```python
from build123d import *

# Parameters (mm, degrees)
F1_DEPTH = 25.4


with BuildPart() as f1:
    # F0 (on Front) → F1 (new body)
    with BuildSketch(Plane.XZ):
        with BuildLine():
            Line((6.3292504433, 31.1127480115), (4.2333333333, 31.4665121818))
            ThreePointArc((4.2333333333, 31.4665121818), (-31.75, 0), (4.2333333333, -31.4665121818))
            Line((4.2333333333, -31.4665121818), (6.3292504433, -31.1127480115))
            ThreePointArc((6.3292504433, -31.1127480115), (24.5867464457, -20.0886634501), (31.75, 0))
            ThreePointArc((31.75, 0), (24.5867464457, 20.0886634501), (6.3292504433, 31.1127480115))
        make_face()
        with BuildLine():
            Line((25.4, 5.588), (25.4, 0))
            Line((25.4, 0), (25.4, -5.588))
            Line((25.4, -5.588), (11.4045717149, -5.588))
            ThreePointArc((11.4045717149, -5.588), (0, -12.7), (-11.4045717149, -5.588))
            Line((-11.4045717149, -5.588), (-25.4, -5.588))
            Line((-25.4, -5.588), (-25.4, 5.588))
            Line((-25.4, 5.588), (-11.4045717149, 5.588))
            ThreePointArc((-11.4045717149, 5.588), (0, 12.7), (11.4045717149, 5.588))
            Line((11.4045717149, 5.588), (25.4, 5.588))
        make_face(mode=Mode.SUBTRACT)
        with BuildLine():
            Line((79.3705518859, 18.7843046381), (6.3292504433, 31.1127480115))
            ThreePointArc((6.3292504433, 31.1127480115), (24.5867464457, 20.0886634501), (31.75, 0))
            Line((31.75, 0), (57.15, 0))
            ThreePointArc((57.15, 0), (63.9015552493, 14.5482217715), (79.3705518859, 18.7843046381))
        make_face()
        with BuildLine():
            ThreePointArc((31.75, 0), (24.5867464457, -20.0886634501), (6.3292504433, -31.1127480115))
            Line((6.3292504433, -31.1127480115), (79.3705518859, -18.7843046381))
            ThreePointArc((79.3705518859, -18.7843046381), (63.9015552493, -14.5482217715), (57.15, 0))
            Line((57.15, 0), (31.75, 0))
        make_face()
        with BuildLine():
            ThreePointArc((95.25, 0), (90.7482217715, 12.2984447507), (79.3705518859, 18.7843046381))
            ThreePointArc((79.3705518859, 18.7843046381), (63.9015552493, 14.5482217715), (57.15, 0))
            ThreePointArc((57.15, 0), (63.9015552493, -14.5482217715), (79.3705518859, -18.7843046381))
            ThreePointArc((79.3705518859, -18.7843046381), (90.7482217715, -12.2984447507), (95.25, 0))
        make_face()
        with BuildLine():
            ThreePointArc((88.9, 0), (76.2, -12.7), (63.5, 0))
            ThreePointArc((63.5, 0), (76.2, 12.7), (88.9, 0))
        make_face(mode=Mode.SUBTRACT)
    extrude(amount=F1_DEPTH)


solid = f1.part
```
Work out the finished part from the listing and answer in its coordinate system (mm). A direction names the side the tool comes from. Round coordinates to 2 decimals unless told otherwise and drop trailing zeros. Write each loop counter-clockwise with the first axis right and the second up, starting at its lowest first coordinate (ties: lowest second). Pieces come first, ordered by that corner, then holes. Notation, with made-up numbers: (27, -7.5) - (57, -7.5) arc R3 cw to (57, -3.5) - close; hole circle Ø3 at (47.5, 22.25). An arc over 180 degrees is marked (long way). Return JSON: item names as keys, results as strings. Group by question number.
Q1. The mould has two halves that part along Z. Classify faces 1 (the cylindrical face through (64.086, -12.522, 3.815)), 2 (the cylindrical face through (-31.74, -12.52, 0.76)), 3 (the flat face through (31, -25.4, 0)): released by +Z, released by -Z, zero draft, split by the parting line, or undercut.
Q2. The part is cut by section B-B on y = -16.25. Write down the section's boundary in (x, z).
Q3. For faces 4 (the flat face through (31, 0, 0)), 5 (the cylindrical face through (-0.2, -12.5, 12.7)), determine the directions among +Z, -Z, +X, -X, +Y, -Y from which every point of the face is accessible in a straight line to the end or side of a thin tool.
Q4. The part is cut by section C-C on x = 76.2. Write down the section's boundary in (y, z), then the cut area to 3 significant figures.
Q5. The part is cut by section A-A on x = 0. Write down the section's boundary in (y, z), then the cut area to 3 significant figures.
Q6. Find the intervals of material crossed by L1, parallel to X at y = -18.5, z = -6; L2, parallel to X at y = -20.5, z = -5; L3, parallel to Z at x = 76.2, y = -7, in increasing order.
Q7. Each of these flat-tipped pins is pushed along its axis until it touches: pin 1 Ø1 at (y, z) = (-12, -18) entering from -X; pin 2 Ø11 at (x, y) = (19.5, -6.5) entering from -Z; pin 3 Ø4 at (x, y) = (-17, -9.5) entering from +Z. Where does it stop, or does it pass through?
Q8. The part is cut by section D-D on x = 47. Write down the section's boundary in (y, z), then the cut area to 3 significant figures.
Solved:
{
 "1": {"face 1": "undercut", "face 2": "split by the parting line", "face 3": "zero draft"},
 "2": {"outline": "(4.23, -31.47) - (79.37, -18.78) arc R19.05 ccw to (79.37, 18.78) - (4.23, 31.47) arc R31.75 ccw (long way) to start; hole (-25.4, -5.59) - (-11.4, -5.59) arc R12.7 ccw to (11.4, -5.59) - (25.4, -5.59) - (25.4, 5.59) - (11.4, 5.59) arc R12.7 ccw to (-11.4, 5.59) - (-25.4, 5.59) - close; hole circle Ø25.4 at (76.2, 0)"},
 "3": {"face 4": "+Z, -Z, +X, -X, +Y", "face 5": "+Y, -Y"},
 "4": {"outline": "(-25.4, -19.32) - (0, -19.32) - (0, -12.7) - (-25.4, -12.7) - close; (-25.4, 12.7) - (0, 12.7) - (0, 19.32) - (-25.4, 19.32) - close", "area": "336 mm²"},
 "5": {"outline": "(-25.4, -31.75) - (0, -31.75) - (0, -12.7) - (-25.4, -12.7) - close; (-25.4, 12.7) - (0, 12.7) - (0, 31.75) - (-25.4, 31.75) - close", "area": "968 mm²"},
 "6": {"L1": "-31.18 to -11.19, 11.19 to 65.01, 87.39 to 94.28", "L2": "-31.35 to -25.4, 25.4 to 64.53, 87.87 to 94.58", "L3": "-19.32 to -12.7, 12.7 to 19.32"},
 "7": {"pin 1": "x = -26.49", "pin 2": "z = -29.82", "pin 3": "z = 27.98"},
 "8": {"outline": "(-25.4, -24.25) - (0, -24.25) - (0, 24.25) - (-25.4, 24.25) - close", "area": "1,230 mm²"}
}
